CAD build for the part. Positions are in the model's coordinates, mm. A direction names the side the tool comes from. Round coordinates to 2 decimals unless told otherwise and drop trailing zeros. Write each loop counter-clockwise with the first axis right and the second up, starting at its lowest first coordinate (ties: lowest second). Pieces come first, ordered by that corner, then holes. Notation, with made-up numbers: (35, 13) - (74, 13) arc R9 ccw to (74, 27) - close; hole circle Ø1 at (30, 20.25). An arc over 180 degrees is marked (long way). Answer in a Markdown table with one row per item.
```python
from build123d import *

# Parameters (mm, degrees)
F1_DEPTH  = 3.175
F3_DEPTH  = 3.176
F5_W      = 1.27
F5_H      = 5.715
F5_W_2    = 5.715
F5_H_2    = 1.27
F6_DEPTH  = 4.445
F7_W      = 1.905
F7_H      = 3.175
F8_DEPTH  = 25.4
F9_W      = 3.175
F9_H      = 1.905
F10_DEPTH = 19.05
F11_R     = 0.9525
F12_DEPTH = 14.9235
F13_R     = 0.254


with BuildPart() as f1:
    # F0 (on Front) → F1 (new body)
    with BuildSketch(Plane.XZ):
        Polygon((2.2225, 10.16), (-2.2225, 10.16), (-2.2225, 2.2225), (-12.7, 2.2225), (-12.7, -2.2225), (-2.2225, -2.2225), (-2.2225, -21.59), (2.2225, -21.59), (2.2225, -2.2225), (12.7, -2.2225), (12.7, 2.2225), (2.2225, 2.2225), align=None)
    extrude(amount=F1_DEPTH)

    # F2 (on Front) → F3 (cut, through all)
    with BuildSketch(Plane.XZ):
        Polygon((-0.9525, -22.86), (0.9525, -22.86), (0.9525, -0.9525), (15.875, -0.9525), (15.875, 0.9525), (0.9525, 0.9525), (0.9525, 22.86), (-0.9525, 22.86), (-0.9525, 0.9525), (-15.875, 0.9525), (-15.875, -0.9525), (-0.9525, -0.9525), align=None)
    extrude(amount=F3_DEPTH, mode=Mode.SUBTRACT)

    # F5 (on offset) → F6 (join)
    with BuildSketch(Plane.XZ.offset(-0.635)):
        with Locations((-8.89, 0)):
            Rectangle(F5_W, F5_H)
        with Locations((8.89, 0)):
            Rectangle(F5_W, F5_H)
        with Locations((0, 6.35)):
            Rectangle(F5_W_2, F5_H_2)
        with Locations((0, -12.7)):
            Rectangle(F5_W_2, F5_H_2)
        with Locations((0, -14.859)):
            Rectangle(F5_W_2, F5_H_2)
        with Locations((0, -17.018)):
            Rectangle(F5_W_2, F5_H_2)
    extrude(amount=F6_DEPTH)

    # F7 (on Top) → F8 (cut, symmetric)
    with BuildSketch(Plane.XY):
        with Locations((0, -1.5875)):
            Rectangle(F7_W, F7_H)
    extrude(amount=F8_DEPTH, both=True, mode=Mode.SUBTRACT)

    # F9 (on Right) → F10 (cut, symmetric)
    with BuildSketch(Plane.YZ):
        with Locations((-1.5875, 0)):
            Rectangle(F9_W, F9_H)
    extrude(amount=F10_DEPTH, both=True, mode=Mode.SUBTRACT)

    # F11 (on face) → F12 (cut, through all)
    with BuildSketch(Plane(origin=(-2.2225, 0, 0), x_dir=(0, -1, 0), z_dir=(-1, 0, 0))):
        with Locations((1.5875, 8.636)):
            Circle(F11_R)
    extrude(amount=-F12_DEPTH, mode=Mode.SUBTRACT)

    # F13
    f13_edges = [f1.edges().sort_by_distance(p)[0] for p in [
        (-2.2225, -0.635, 8.636),
        (2.2225, -0.635, 8.636),
    ]]
    fillet(f13_edges, radius=F13_R)


solid = f1.part
```
Q1. Drill centre lines: line 1 (Z direction, x = -1.5, y = 0.15) (3 decimals); line 2 (X direction, y = -1.75, z = -1); line 3 (X direction, y = -0.05, z = 3). Where is each one in solid material? Low to high.
Computed:
| item | result |
|---|---|
| line 1 | z = -17.653 to -16.383, -15.494 to -14.224, -13.335 to -12.065, 5.715 to 6.985 |
| line 2 | x = -12.7 to -0.95, 0.95 to 12.7 |
| line 3 | x = -2.22 to -0.95, 0.95 to 2.22 |
Q2. 3-axis set-ups, long thin cutter, end or side, ignore diameter. For faces 5 (the flat face through (0, 0.4, -16.383)), 6 (the flat face through (-9, 0, 0)), 7 (the flat face through (11, -3.175, 2)): which of +Z, -Z, +X, -X, +Y, -Y reach the whole face in a straight line?
Computed:
| item | result |
|---|---|
| face 5 | none |
| face 6 | +X, -X |
| face 7 | +Z, -Z, +X, -Y |
Q3. Saw through at D-D on z = -17. List the corners of the cut face in (x, y) (1 decimal), then the cut area to 3 significant figures.
Computed:
| item | result |
|---|---|
| outline | (-2.9, -3.8) - (2.9, -3.8) - (2.9, 0.6) - (-2.9, 0.6) - close; hole (-1, -3.2) - (1, -3.2) - (1, 0) - (-1, 0) - close |
| area | 19.4 mm2 |
Q4. Saw through at A-A on z = -10. List the corners of the cut face in (x, y) (1 decimal), then the cut area to 3 significant figures.
Computed:
| item | result |
|---|---|
| outline | (-2.2, -3.2) - (-1, -3.2) - (-1, 0) - (-2.2, 0) - close; (1, -3.2) - (2.2, -3.2) - (2.2, 0) - (1, 0) - close |
| area | 8.06 mm2 |
Q5. Saw through at B-B on x = -7.75. List the corners of the cut face in (y, z) (1 decimal).
Computed:
| item | result |
|---|---|
| outline | (-3.2, -2.2) - (0, -2.2) - (0, -1) - (-3.2, -1) - close; (-3.2, 1) - (0, 1) - (0, 2.2) - (-3.2, 2.2) - close |
Q6. Pull direction X, two halves, no side cores. Call faces 1 (the flat face through (2, -3.175, -5)), 2 (the flat face through (11, -2, 2.222)), 3 (the flat face through (-2.222, -2, -16)), 4 (the flat face through (-5, -2, 2.222)): released by +X, released by -X, zero draft, split by the parting line, or undercut.
Computed:
| item | result |
|---|---|
| face 1 | undercut |
| face 2 | zero draft |
| face 3 | released by -X |
| face 4 | undercut |
Q7. Saw through at C-C on x = 9. List the corners of the cut face in (y, z) (1 decimal), then the cut area to 3 significant figures.
Computed:
| item | result |
|---|---|
| outline | (-3.8, -2.9) - (0.6, -2.9) - (0.6, 2.9) - (-3.8, 2.9) - close; hole (-3.2, -1) - (0, -1) - (0, 1) - (-3.2, 1) - close |
| area | 19.4 mm2 |
Q8. Flat gauge pins, fed straight in: pin 1 (1 mm diameter, centred on y = -1.5, z = -14.5, fed in from -X); pin 2 (1.4 mm diameter, centred on x = 1.5, z = -20, fed in from -Y) (3 decimals); pin 3 (1.5 mm diameter, centred on y = -1.59, z = 8.64, fed in from -X); pin 4 (1.5 mm diameter, centred on y = -2, z = -8.5, fed in from -X). Where does each tip first touch, or does it go through?
Computed:
| item | result |
|---|---|
| pin 1 | stops at x = -2.86 |
| pin 2 | stops at y = -3.175 |
| pin 3 | passes through |
| pin 4 | stops at x = -2.22 |
